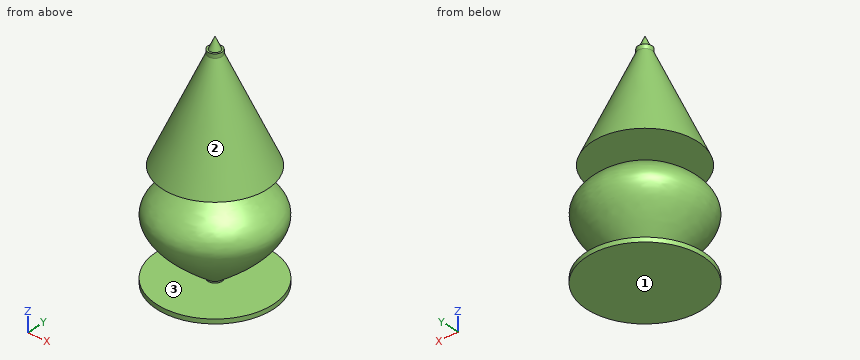
```python
from build123d import *

# Parameters (mm, degrees)
F0_R     = 3.3510634676
F2_DEPTH = 50
F7_W     = 27.5042355061
F7_H     = 2.1134242415


with BuildPart() as f2:
    # F0 (on Top) → F2 (new body, symmetric)
    with BuildSketch(Plane.XY):
        Circle(F0_R)
    extrude(amount=F2_DEPTH, both=True)

    # F3 (on Right) → F4 (revolve)
    with BuildSketch(Plane.YZ):
        Polygon((0, 0), (0, 55.571809411), (-24.8537249863, 0), align=None)
    revolve(axis=Axis((0, 0, 27.7859047055), (0, 0, -1)))

    # F5 (on Right) → F6 (revolve)
    with BuildSketch(Plane.YZ):
        with BuildLine():
            Line((0, -50.3720380366), (0, 0))
            add(Edge.make_bspline(
                [(0, 0), (-13.3377713463, -6.1965659051), (-41.2377708413, -19.1585654127), (-14.1423062486, -39.6675193412), (0, -50.3720380366)],
                knots=[0, 0, 0, 0, 0.4780563293, 1, 1, 1, 1], degree=3))
        make_face()
    revolve(axis=Axis((0, 0, -25.1860190183), (0, 0, -1)))

    # F7 (on Right) → F8 (revolve)
    with BuildSketch(Plane.YZ):
        with Locations((13.752117753, -49.5501495898)):
            Rectangle(F7_W, F7_H)
    revolve(axis=Axis((0, 0, -49.5501495898), (0, 0, 1)))


solid = f2.part
```
Build history of the part. All positions in model axes, mm. Face numbers are marked on the shaded views. Give positions to 0.01 mm unless a question says otherwise; leave off trailing zeros. Loops run counter-clockwise (first coordinate to the right, second up) from the corner with the lowest first, then second, coordinate; pieces in that order, holes last.
1) Two-plate mould, pull along Z, no slides. Class the marked faces 1, 2 and 3: released by +Z, released by -Z, zero draft, split by the parting line, or undercut.
Values follow:
face 1: released by -Z
face 2: released by +Z
face 3: undercut
2) Band-saw the part on C-C on z = 39. List the corners of the cut face in (x, y).
Values follow:
outline: circle Ø14.82 at (0, 0)
3) Drop flat-ended pins along their axis: P1, Ø3, axis at x = -7.5, z = 31.5, coming from the +Y side; P2, Ø10, axis at y = -15.5, z = -29, coming from the -X side; P3, Ø6, axis at x = -3, y = -17, coming from the +Z side. Give the stop position or say it passes through.
Values follow:
P1: stops at y = 9.22
P2: stops at x = -23.53
P3: stops at z = 23.68
4) Band-saw the part on A-A on y = 5.5. State how many separate pieces and enclosed holes the cut face has, then the cut area to 3 significant figures.
Values follow:
separate pieces: 3
enclosed holes: 0
area: 2,920 mm2
5) Probe line 1 along Z through (x, y) = (8, 0); line 2 along Z through (x, y) = (4.5, -8); line 3 along Z through (x, y) = (17, 19.5). List the from-to ranges inside material, lowest first.
Values follow:
line 1: z = -50.61 to -48.49, -44.25 to -3.78, 0 to 37.68
line 2: z = -50.61 to -48.49, -43.33 to -4.36, 0 to 35.05
line 3: z = -50.61 to -48.49, -26.51 to -16.18
